from build123d import *

# Parameters (mm, degrees)
SKETCH_2_W               = 117.5
SKETCH_2_H               = 180
EXTRUDE_2_DEPTH          = 3
EXTRUDE_5_DEPTH          = 6
EXTRUDE_START            = -6
EXTRUDE_6_DEPTH          = 6
EXTRUDE_8_DEPTH          = 8
CUT_EXTRUDE_1_DEPTH      = 188
CUT_EXTRUDE_1_DEPTH_BACK = 20
SKETCH_8_R               = 2.5
FILLET_1_R               = 3
SKETCH_10_W              = 6
SKETCH_10_H              = 168
EXTRUDE_9_DEPTH          = 45
CUT_EXTRUDE_2_DEPTH      = 159.688767718
SKETCH_12_W              = 3
SKETCH_12_H              = 20
EXTRUDE_10_DEPTH         = 10


with BuildPart() as part:
    # 草圖2 → 填料-伸長2 (new body)
    with BuildSketch(Plane.XY):
        Rectangle(SKETCH_2_W, SKETCH_2_H)
    extrude(amount=EXTRUDE_2_DEPTH)

    # 草圖4 → 填料-伸長5 (add)
    with BuildSketch(Plane.XZ.offset(90)):
        with BuildLine():
            Line((-58.75, 3), (-58.75, 58))
            ThreePointArc((-58.75, 58), (0, 116.75), (58.75, 58))
            Line((58.75, 58), (58.75, 3))
            Line((58.75, 3), (-58.75, 3))
        make_face()
    extrude(amount=-EXTRUDE_5_DEPTH)

    # 草圖5 → 填料-伸長6 (add)
    with BuildSketch(Plane(origin=(0, 90, 0), x_dir=(1, 0, 0), z_dir=(0, 1, 0)).offset(EXTRUDE_START)):
        with BuildLine():
            Line((-58.75, -3), (-58.75, -58))
            ThreePointArc((-58.75, -58), (0, -116.75), (58.75, -58))
            Line((58.75, -58), (58.75, -3))
            Line((58.75, -3), (-58.75, -3))
        make_face()
    extrude(amount=EXTRUDE_6_DEPTH)

    # 草圖7 → 填料-伸長8 (add)
    with BuildSketch(Plane.ZY.offset(58.75)):
        Polygon((3, 84), (58, 84), (58, 79), (48, 79), (48, -79), (58, -79), (58, -84), (3, -84), align=None)
    extrude(amount=-EXTRUDE_8_DEPTH)

    # 草圖8 → 除料-伸長1 (cut, two sides: drawn at the far end of the back side and taken through both)
    with BuildSketch(Plane.XZ.offset(-79).offset(-CUT_EXTRUDE_1_DEPTH_BACK)):
        with Locations(Location((-54.75, 53, 0), (0, 0, 90))):
            Circle(SKETCH_8_R)
    extrude(amount=CUT_EXTRUDE_1_DEPTH + CUT_EXTRUDE_1_DEPTH_BACK, mode=Mode.SUBTRACT)

    # 圓角1
    fillet_1_edges = [part.edges().sort_by_distance(p)[0] for p in [
        (-58.75, -81.5, 58),
        (-58.75, 81.5, 58),
    ]]
    fillet(fillet_1_edges, radius=FILLET_1_R)

    # 草圖10 → 填料-伸長9 (add)
    with BuildSketch(Plane.XY.offset(3)):
        with Locations((55.75, 0)):
            Rectangle(SKETCH_10_W, SKETCH_10_H)
    extrude(amount=EXTRUDE_9_DEPTH)

    # 草圖11 → 除料-伸長2 (cut, through all)
    with BuildSketch(Plane(origin=(0, 0, 0), x_dir=(-1, 0, 0), z_dir=(0, 0, -1))):
        with BuildLine():
            Line((2.75, 8.745412879), (2.75, -7.754587121))
            ThreePointArc((2.75, -7.754587121), (0, -10.504587121), (-2.75, -7.754587121))
            Line((-2.75, -7.754587121), (-2.75, 8.745412879))
            ThreePointArc((-2.75, 8.745412879), (0, 11.495412879), (2.75, 8.745412879))
        make_face()
    extrude(amount=-CUT_EXTRUDE_2_DEPTH, mode=Mode.SUBTRACT)

    # 草圖12 → 填料-伸長10 (add)
    with BuildSketch(Plane(origin=(58.75, 0, 0), x_dir=(0, 0, -1), z_dir=(1, 0, 0))):
        with Locations((-46.5, 0)):
            Rectangle(SKETCH_12_W, SKETCH_12_H)
    extrude(amount=EXTRUDE_10_DEPTH)


solid = part.part
Geometry check sheet. Reference: the model listing, model coordinates, mm. A direction names the side the tool comes from. Coordinates: 2 decimals unless noted, no trailing zeros. Write each loop counter-clockwise with the first axis right and the second up, starting at its lowest first coordinate (ties: lowest second). Pieces come first, ordered by that corner, then holes. Notation, with made-up numbers: (13, -20) -> (66, -20) arc R23 cw to (66, -1) -> close; hole circle Ø2 at (47, -22.75). An arc over 180 degrees is marked (long way). One line per question, with ' | ' between items.
1. Cross-section at D-D on z = 31.5. Record the cut outline in (x, y), and give its area (3 significant figures).
Answers:
outline: (-58.75, -90) -> (58.75, -90) -> (58.75, 90) -> (-58.75, 90) -> close; hole (-50.75, -84) -> (52.75, -84) -> (52.75, 84) -> (-50.75, 84) -> close | area: 3,760 mm²
2. Thickness scan on probe 1 along Y at (x, z) = (-2.5, 71); probe 2 along X at (y, z) = (82.5, 53); probe 3 along X at (y, z) = (65, 29). Record the ranges inside material, lowest first. Write a range as from..to.
Answers:
probe 1: y = -90..-84, 84..90 | probe 2: x = -58.75..-57.25, -52.25..-50.75 | probe 3: x = -58.75..-50.75, 52.75..58.75
3. Cross-section at C-C on y = -0.5. Record the cut outline in (x, z).
Answers:
outline: (-58.75, 0) -> (-2.75, 0) -> (-2.75, 3) -> (-50.75, 3) -> (-50.75, 48) -> (-58.75, 48) -> close; (2.75, 0) -> (58.75, 0) -> (58.75, 45) -> (68.75, 45) -> (68.75, 48) -> (52.75, 48) -> (52.75, 3) -> (2.75, 3) -> close
4. Cross-section at A-A on z = 53. Record the cut outline in (x, y).
Answers:
outline: (-58.75, -90) -> (-57.25, -90) -> (-57.25, -79) -> (-58.75, -79) -> close; (-58.75, 79) -> (-57.25, 79) -> (-57.25, 90) -> (-58.75, 90) -> close; (-52.25, -90) -> (58.75, -90) -> (58.75, -84) -> (-50.75, -84) -> (-50.75, -79) -> (-52.25, -79) -> close; (-52.25, 79) -> (-50.75, 79) -> (-50.75, 84) -> (58.75, 84) -> (58.75, 90) -> (-52.25, 90) -> close
5. Set-up check for faces 1 (the flat face through (-11, 1, 3)), 2 (the cylindrical face through (-53.79, 84.58, 55.31)), 3 (the flat face through (64, 0, 45)), 4 (the flat face through (-52, -79, 53)), 5 (the flat face through (12, 1, 0)): record each of +Z, -Z, +X, -X, +Y, -Y from which the full face is reachable in a straight line by a thin tool's end or side.
Answers:
face 1: +Z | face 2: +Y, -Y | face 3: -Z, +X, +Y, -Y | face 4: +Z, +X, -X | face 5: -Z, +X, -X, +Y, -Y
6. Cross-section at B-B on x = 0. Record the cut outline in (y, z).
Answers:
outline: (-90, 0) -> (-10.5, 0) -> (-10.5, 3) -> (-84, 3) -> (-84, 116.75) -> (-90, 116.75) -> close; (11.5, 0) -> (90, 0) -> (90, 116.75) -> (84, 116.75) -> (84, 3) -> (11.5, 3) -> close
7. Draft check along X on faces 6 (the flat face through (-55, 1, 48)), 7 (the flat face through (-50.75, 1, 25)), 8 (the cylindrical face through (-1.292, 86.958, 116.736)). Enter one of: +X half, -X half, draft (parallel to the pull), parting line (faces both ways), or undercut.
Answers:
face 6: draft | face 7: undercut | face 8: parting line
8. Depth check by flat-ended pin: pin 1 Ø13 at (x, y) = (62, -36.5) entering from +Z; pin 2 Ø0.9 at (x, z) = (62.5, 46) entering from +Y; pin 3 Ø4 at (y, z) = (-7, 30) entering from +X. Enter the tip coordinate at first touch or a pass-through.
Answers:
pin 1: stops at z = 48 | pin 2: stops at y = 10 | pin 3: stops at x = 58.75
